Could you check a few things on this drawing? It's one solid part, dimensions in mm from its lowest x, y, z. Round coordinates to 2 decimals unless told otherwise and drop trailing zeros. Order: outer loops, then holes, each group sorted by start corner. A loop starts at its lowest first (then second) coordinate and runs counter-clockwise, first axis right, second up. Notation, with made-up numbers: (69.5, 79) -> (110.5, 79) arc R11 cw to (110.5, 89) -> close; hole circle Ø8 at (-22, 35.25). An arc over 180 degrees is marked (long way). Use a Markdown table: item, result. Add a question column.
(1) I'm going to push flat-ended pins straight in: P1, Ø1.5, axis at y = 76.5, z = 1.5, coming from the +X side; P2, Ø0.9, axis at x = 27.5, z = 1, coming from the -Y side; P3, Ø1.5, axis at y = 3, z = 1, coming from the -X side. Where does each tip first touch, or does it pass through?
(2) I want a section at B-B, the plane y = 38.5. Please give me the cut outline in (x, z).
(3) I want a section at A-A, the plane x = 29.5. Please give me the cut outline in (y, z) (1 decimal), then the cut area to 3 significant figures.
(4) I want a section at D-D, the plane x = 5. Please give me the cut outline in (y, z) (1 decimal), then the cut area to 3 significant figures.
(5) If I drill on probe 1 along Y at (x, z) = (28.5, 2.35) (1 decimal); probe 2 along Y at (x, z) = (16, 0.55) (1 decimal); probe 3 along Y at (x, z) = (14.5, 2.8), over which ranges is the centre line in solid material (lowest first)?
(6) I want a section at C-C, the plane y = 50.5. Please give me the cut outline in (x, z).
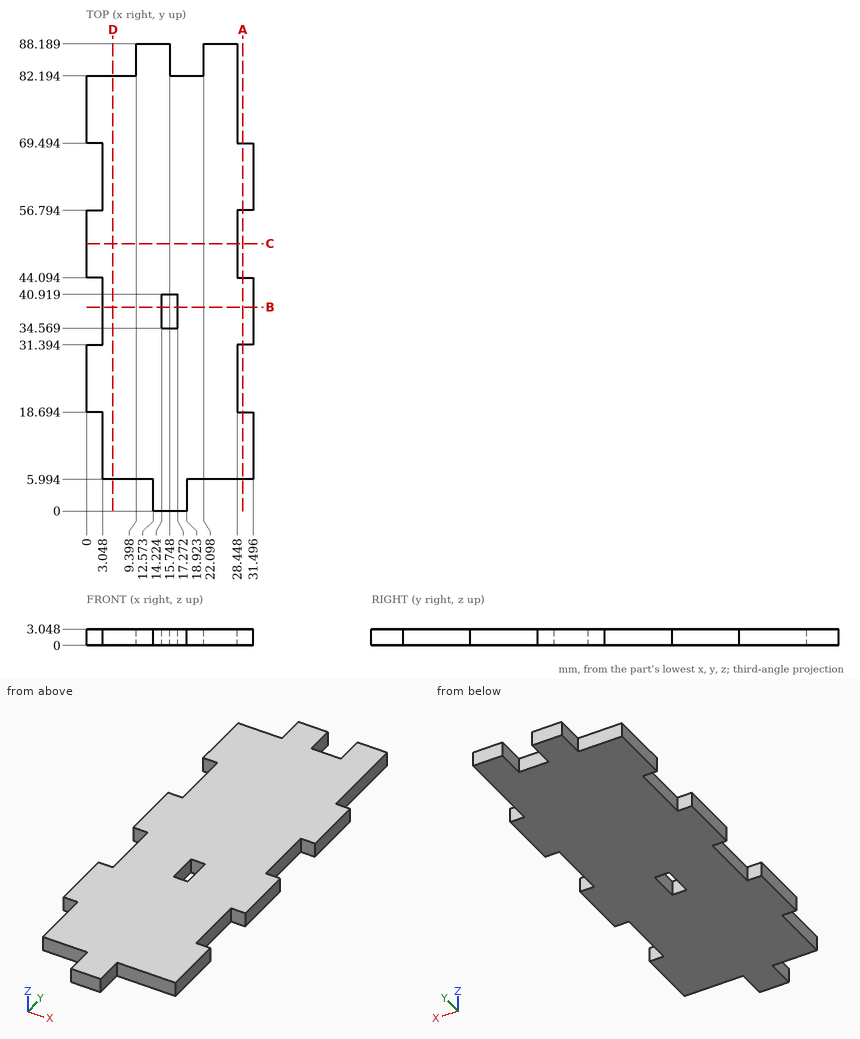
Taken from the geometry:
| question | item | result |
|---|---|---|
| 1 | P1 | stops at x = 28.45 |
| 1 | P2 | stops at y = 5.99 |
| 1 | P3 | stops at x = 12.57 |
| 2 | outline | (3.05, 0) -> (14.22, 0) -> (14.22, 3.05) -> (3.05, 3.05) -> close; (17.27, 0) -> (31.5, 0) -> (31.5, 3.05) -> (17.27, 3.05) -> close |
| 3 | outline | (6, 0) -> (18.7, 0) -> (18.7, 3) -> (6, 3) -> close; (31.4, 0) -> (44.1, 0) -> (44.1, 3) -> (31.4, 3) -> close; (56.8, 0) -> (69.5, 0) -> (69.5, 3) -> (56.8, 3) -> close |
| 3 | area | 116 mm2 |
| 4 | outline | (6, 0) -> (82.2, 0) -> (82.2, 3) -> (6, 3) -> close |
| 4 | area | 232 mm2 |
| 5 | probe 1 | y = 6 to 18.7, 31.4 to 44.1, 56.8 to 69.5 |
| 5 | probe 2 | y = 0 to 34.6, 40.9 to 82.2 |
| 5 | probe 3 | y = 0 to 34.57, 40.92 to 88.19 |
| 6 | outline | (0, 0) -> (28.45, 0) -> (28.45, 3.05) -> (0, 3.05) -> close |
